Work out the finished part from the listing and answer in its coordinate system (mm). Face numbers are marked on the shaded views. A direction names the side the tool comes from. Round coordinates to 2 decimals unless told otherwise and drop trailing zeros. Order: outer loops, then holes, each group sorted by start corner. A loop starts at its lowest first (then second) coordinate and runs counter-clockwise, first axis right, second up. Notation, with made-up numbers: (-13.5, 37.25) -> (-8.5, 37.25) arc R28 cw to (-8.5, 75.25) -> close; hole circle Ø10 at (-38, 79.25). An arc over 180 degrees is marked (long way). Use a Markdown table: item, result. Add a question column.
Item 1: A tool of negligible diameter and unlimited length cuts with its end or side. For the marked faces 1, 2 and 3, from which of +Z, -Z, +X, -X, +Y, -Y can it reach the whole face along a straight path? Write none if from no direction.
Item 2: Flat-ended cylindrical pins translate along their axes: P1, Ø2.5, axis at x = -0.5, y = -2, coming from the -Z side; P2, Ø0.9, axis at x = 0.5, y = -3, coming from the +Z side; P3, Ø3, axis at x = -2, z = 2.5, coming from the +Y side; P4, Ø4, axis at x = 0, y = 8, coming from the +Z side. Find the tip coordinate at first contact, or state that the pin passes through.
Item 3: Find the intervals of material crossed by L1, parallel to Y at x = -2.5, z = 0; L2, parallel to Z at x = 0, y = 11; L3, parallel to Y at x = 2, z = -4.25, in increasing order. Write a range as [from, to].
Item 4: For a pull along Z with two mould halves and no side action, classify the marked faces 4, 5 and 6 as +Z half, -Z half, draft (parallel to the pull), parting line (faces both ways), or undercut.
Item 5: A cutting plane is placed at A-A, the plane x = 0.5. Give the number of separate pieces and of enclosed holes in the cut face, plus the area to 3 significant figures.
Item 6: A cutting plane is placed at B-B, the plane y = -3.5. Determine the outline of the cut face in (x, z).
Item 7: A cutting plane is placed at D-D, the plane y = 8. Determine the outline of the cut face in (x, z).
from build123d import *

# Parameters (mm, degrees)
SKETCH1_W           = 9.5
SKETCH1_H           = 12
BOSS_EXTRUDE1_DEPTH = 12
SKETCH2_W           = 13
SKETCH2_H           = 5
CUT_EXTRUDE1_DEPTH  = 10
SKETCH3_R           = 2.38125
CUT_EXTRUDE2_DEPTH  = 18.622783549
CUT_EXTRUDE3_START  = -13
CUT_EXTRUDE3_DEPTH  = 31.622783549
SKETCH6_W           = 9.5
SKETCH6_H           = 8
BOSS_EXTRUDE3_DEPTH = 8
SKETCH7_R           = 1
CUT_EXTRUDE5_DEPTH  = 10
FILLET2_R           = 4
FILLET3_START       = -6
FILLET3_DEPTH       = 12
FILLET3_START_2     = -4.75
FILLET3_2_DEPTH     = 9.5


with BuildPart() as part:
    # Sketch1 → Boss-Extrude1 (new body)
    with BuildSketch(Plane(origin=(0, 0, 0), x_dir=(1, 0, 0), z_dir=(0, 1, 0))):
        Rectangle(SKETCH1_W, SKETCH1_H)
    extrude(amount=BOSS_EXTRUDE1_DEPTH)

    # Sketch2 → Cut-Extrude1 (cut)
    with BuildSketch(Plane(origin=(0, 12, 0), x_dir=(1, 0, 0), z_dir=(0, 1, 0))):
        Rectangle(SKETCH2_W, SKETCH2_H)
    extrude(amount=-CUT_EXTRUDE1_DEPTH, mode=Mode.SUBTRACT)

    # Sketch3 → Cut-Extrude2 (cut, through all)
    with BuildSketch(Plane(origin=(0, 0, -6), x_dir=(-1, 0, 0), z_dir=(0, 0, -1))):
        with Locations((0, 8)):
            Circle(SKETCH3_R)
    extrude(amount=-CUT_EXTRUDE2_DEPTH, mode=Mode.SUBTRACT)

    # Sketch4 → Cut-Extrude3 (cut)
    with BuildSketch(Plane(origin=(0, 0, -6), x_dir=(-1, 0, 0), z_dir=(0, 0, -1)).offset(CUT_EXTRUDE3_START)):
        with BuildLine():
            Line((-4.75, 12), (-4.75, 7.25))
            ThreePointArc((-4.75, 7.25), (-3.358757211, 10.608757211), (0, 12))
            Line((0, 12), (-4.75, 12))
        make_face()
    cut_extrude3 = extrude(amount=CUT_EXTRUDE3_DEPTH, mode=Mode.SUBTRACT)

    # Mirror1: Cut-Extrude3 across plane
    add(cut_extrude3.mirror(Plane(origin=(0, 0, 0), x_dir=(0, 0, 1), z_dir=(1, 0, 0))), mode=Mode.SUBTRACT)

    # Sketch6 → Boss-Extrude3 (add)
    with BuildSketch(Plane.XZ):
        Rectangle(SKETCH6_W, SKETCH6_H)
    extrude(amount=BOSS_EXTRUDE3_DEPTH)

    # Sketch7 → Cut-Extrude5 (cut)
    with BuildSketch(Plane.ZY.offset(4.75)):
        with Locations((0, -4)):
            Circle(SKETCH7_R)
    extrude(amount=-CUT_EXTRUDE5_DEPTH, mode=Mode.SUBTRACT)

    # Fillet2
    fillet2_edges = [part.edges().sort_by_distance(p)[0] for p in [
        (0, -8, 4),
        (0, -8, -4),
    ]]
    fillet(fillet2_edges, radius=FILLET2_R - 0.0001)  # a hair under: the kernel refuses the full size

    # Fillet3: read off the stored shape, not the designer's step
    # Fillet3 outline → Fillet3 (cut)
    with BuildSketch(Plane.YZ.offset(FILLET3_START)):
        with BuildLine():
            Line((0, 6), (0, 5))
            ThreePointArc((0, 5), (0.292893219, 5.707106781), (1, 6))
            Line((1, 6), (0, 6))
        make_face()
        with BuildLine():
            ThreePointArc((1, -6), (0.292893219, -5.707106781), (0, -5))
            Line((0, -5), (0, -6))
            Line((0, -6), (1, -6))
        make_face()
    extrude(amount=FILLET3_DEPTH, mode=Mode.SUBTRACT)

    # Fillet3 2 outline → Fillet3 2 (add)
    with BuildSketch(Plane.YZ.offset(FILLET3_START_2)):
        with BuildLine():
            Line((0, 4), (0, 5))
            ThreePointArc((0, 5), (-0.292893219, 4.292893219), (-1, 4))
            Line((-1, 4), (0, 4))
        make_face()
        with BuildLine():
            ThreePointArc((-1, -4), (-0.292893219, -4.292893219), (0, -5))
            Line((0, -5), (0, -4))
            Line((0, -4), (-1, -4))
        make_face()
    extrude(amount=FILLET3_2_DEPTH)


solid = part.part
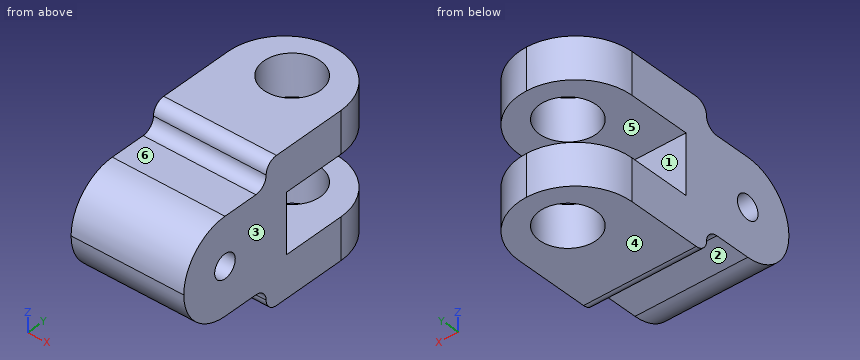
Reported:
| question | item | result |
|---|---|---|
| 1 | face 1 | +X, -X, +Y |
| 1 | face 2 | -Z, +X, -X, -Y |
| 1 | face 3 | +Z, -Z, +X, +Y, -Y |
| 2 | P1 | z = -4.03 |
| 2 | P2 | z = 4 |
| 2 | P3 | y = 11.97 |
| 2 | P4 | through |
| 3 | L1 | [-8, -5], [-3, 2] |
| 3 | L2 | [-6, -2.5], [2.5, 6] |
| 3 | L3 | [-0.34, 6.71], [9.29, 11.56] |
| 4 | face 4 | -Z half |
| 4 | face 5 | undercut |
| 4 | face 6 | +Z half |
| 5 | separate pieces | 3 |
| 5 | enclosed holes | 1 |
| 5 | area | 115 mm² |
| 6 | outline | (-4.75, -4) -> (4.75, -4) -> (4.75, -0.87) -> (-4.75, -0.87) -> close; (-4.75, 0.87) -> (4.75, 0.87) -> (4.75, 4) -> (-4.75, 4) -> close |
| 7 | outline | (-4.69, -6) -> (-2.38, -6) -> (-2.38, -2.5) -> (-4.69, -2.5) -> close; (-4.69, 2.5) -> (-2.38, 2.5) -> (-2.38, 6) -> (-4.69, 6) -> close; (2.38, -6) -> (4.69, -6) -> (4.69, -2.5) -> (2.38, -2.5) -> close; (2.38, 2.5) -> (4.69, 2.5) -> (4.69, 6) -> (2.38, 6) -> close |
